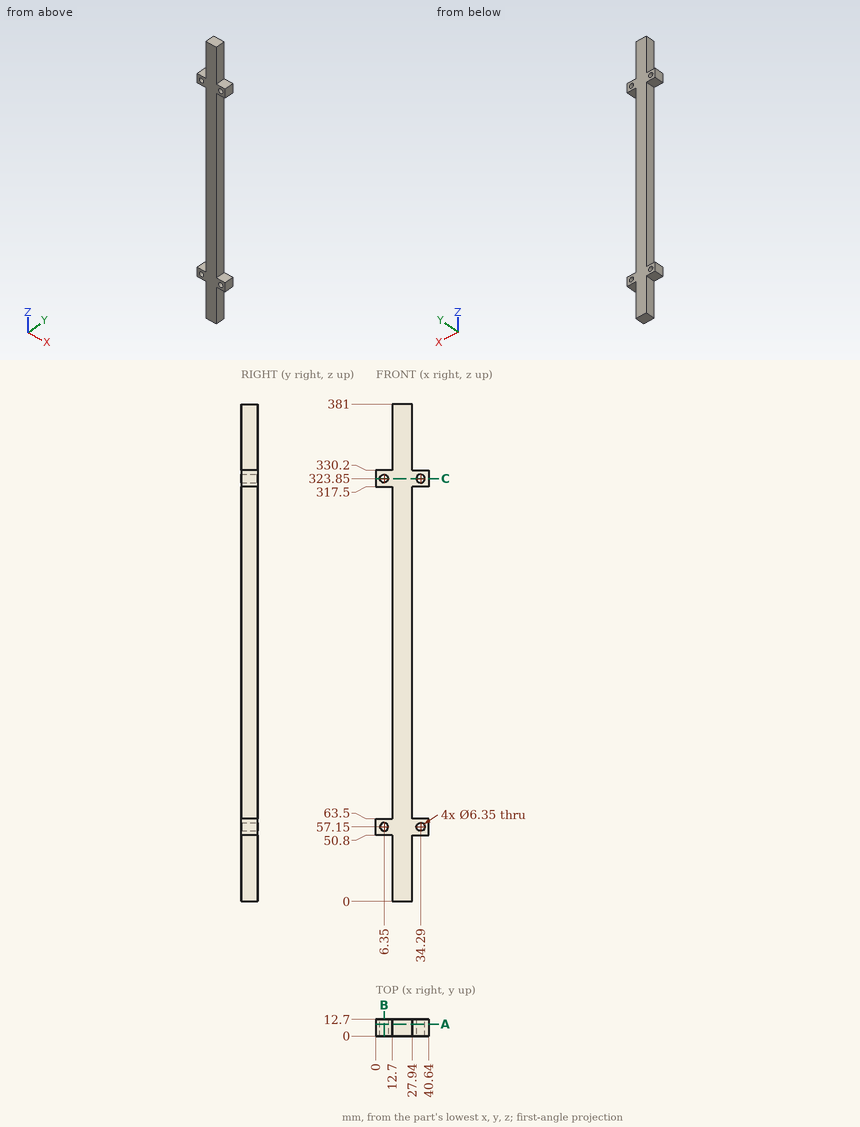
Design review of the part shown in the three views and the two pictorial views. Dimensions are in mm from the part's minimum x, y and z. Round coordinates to 2 decimals unless told otherwise and drop trailing zeros. Write each loop counter-clockwise with the first axis right and the second up, starting at its lowest first coordinate (ties: lowest second). Pieces come first, ordered by that corner, then holes. Notation, with made-up numbers: (-30.5, 40) -> (5.5, 40) arc R18 ccw to (5.5, 64) -> close; hole circle Ø3 at (31.5, 16.5). An arc over 180 degrees is marked (long way). One line per question, with ' | ' between items. Start each with the question number.
1) Add section C-C (z = 323.85). Write out the cut boundary in (x, y) (3 decimals), and give its area (3 significant figures).
2) Wall thickness on line 1 along Z through (x, y) = (6.35, 8) (3 decimals); line 2 along X through (y, z) = (7, 323.85) (3 decimals); line 3 along Z through (x, y) = (5, 10): over which ranges is each line inside the solid? List them lowest first.
3) Add section A-A (y = 9). Write out the cut boundary in (x, z) (3 decimals), and give its area (3 significant figures).
4) For pin 1 Ø4 at (x, y) = (35.5, 8) entering from -Z; pin 2 Ø1 at (y, z) = (4.5, 212.5) entering from +X; pin 3 Ø6.5 at (y, z) = (9, 190) entering from -X, all flat-tipped, find the tip position at first contact; note any pin that passes through.
5) Add section B-B (x = 6.35). Write out the cut boundary in (y, z) (3 decimals), and give its area (3 significant figures).
Reported:
1) outline: (0, 0) -> (3.175, 0) -> (3.175, 12.7) -> (0, 12.7) -> close; (9.525, 0) -> (31.115, 0) -> (31.115, 12.7) -> (9.525, 12.7) -> close; (37.465, 0) -> (40.64, 0) -> (40.64, 12.7) -> (37.465, 12.7) -> close | area: 355 mm²
2) line 1: z = 50.8 to 53.975, 60.325 to 63.5, 317.5 to 320.675, 327.025 to 330.2 | line 2: x = 0 to 3.175, 9.525 to 31.115, 37.465 to 40.64 | line 3: z = 50.8 to 54.28, 60.02 to 63.5, 317.5 to 320.98, 326.72 to 330.2
3) outline: (0, 50.8) -> (12.7, 50.8) -> (12.7, 0) -> (27.94, 0) -> (27.94, 50.8) -> (40.64, 50.8) -> (40.64, 63.5) -> (27.94, 63.5) -> (27.94, 317.5) -> (40.64, 317.5) -> (40.64, 330.2) -> (27.94, 330.2) -> (27.94, 381) -> (12.7, 381) -> (12.7, 330.2) -> (0, 330.2) -> (0, 317.5) -> (12.7, 317.5) -> (12.7, 63.5) -> (0, 63.5) -> close; hole circle Ø6.35 at (6.35, 57.15); hole circle Ø6.35 at (6.35, 323.85); hole circle Ø6.35 at (34.29, 57.15); hole circle Ø6.35 at (34.29, 323.85) | area: 6,320 mm²
4) pin 1: stops at z = 50.8 | pin 2: stops at x = 27.94 | pin 3: stops at x = 12.7
5) outline: (0, 50.8) -> (12.7, 50.8) -> (12.7, 53.975) -> (0, 53.975) -> close; (0, 60.325) -> (12.7, 60.325) -> (12.7, 63.5) -> (0, 63.5) -> close; (0, 317.5) -> (12.7, 317.5) -> (12.7, 320.675) -> (0, 320.675) -> close; (0, 327.025) -> (12.7, 327.025) -> (12.7, 330.2) -> (0, 330.2) -> close | area: 161 mm²
